Verification items for the finished model (mm, model axes). Round coordinates to 2 decimals unless told otherwise and drop trailing zeros. Write each loop counter-clockwise with the first axis right and the second up, starting at its lowest first coordinate (ties: lowest second). Pieces come first, ordered by that corner, then holes.
from build123d import *

# Parameters (mm, degrees)
SKETCH_W            = 19.36
SKETCH_H            = 103.56
PAD_DEPTH           = 0.8
POCKET_DEPTH        = 5
LINEARPATTERN_COUNT = 6
LINEARPATTERN_PITCH = 16.84


with BuildPart() as part:
    # Sketch → Pad (new body)
    with BuildSketch(Plane.XY):
        with Locations((-9.68, 51.78)):
            Rectangle(SKETCH_W, SKETCH_H)
    extrude(amount=PAD_DEPTH)

    # Sketch001 (on Face6 of Pad) → Pocket (cut)
    with BuildSketch(Plane.XY.offset(0.8)):
        with BuildLine():
            Line((-17.68, 16.68), (-17.68, 2.68))
            ThreePointArc((-17.68, 2.68), (-17.387107, 1.972893), (-16.68, 1.68))
            Line((-16.68, 1.68), (-2.68, 1.68))
            ThreePointArc((-2.68, 1.68), (-1.972893, 1.972893), (-1.68, 2.68))
            Line((-1.68, 2.68), (-1.68, 16.68))
            ThreePointArc((-1.68, 16.68), (-1.972893, 17.387107), (-2.68, 17.68))
            Line((-2.68, 17.68), (-16.68, 17.68))
            ThreePointArc((-16.68, 17.68), (-17.387107, 17.387107), (-17.68, 16.68))
        make_face()
    pocket = extrude(amount=-POCKET_DEPTH, mode=Mode.SUBTRACT)

    # LinearPattern: Pocket ×6
    with Locations(*[(0, i * LINEARPATTERN_PITCH, 0) for i in range(1, LINEARPATTERN_COUNT)]):
        add(pocket, mode=Mode.SUBTRACT)


solid = part.part
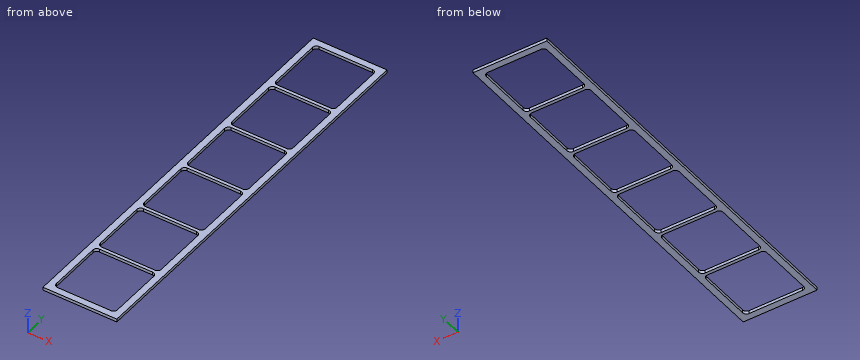
Q1. Sectioned sample at A-A (y = 72). Enter the section's corners in (x, z), plus the area to 3 significant figures.
Recorded:
outline: (-19.36, 0) - (-17.68, 0) - (-17.68, 0.8) - (-19.36, 0.8) - close; (-1.68, 0) - (0, 0) - (0, 0.8) - (-1.68, 0.8) - close
area: 2.69 mm2
Q2. Sectioned sample at C-C (z = 0.3). Give the number of separate pieces and of enclosed holes in the cut face, plus the area to 3 significant figures.
Recorded:
separate pieces: 1
enclosed holes: 6
area: 474 mm2
Q3. Depth check by flat-ended pin: P1, Ø5, axis at x = -4.5, y = 88, coming from the +Z side. Enter the tip coordinate at first touch or a pass-through.
Recorded:
P1: stops at z = 0.8
Q4. Material ranges on line 1 along X through (y, z) = (11.5, 0.6), recorded low to high.
Recorded:
line 1: x = -19.36 to -17.68, -1.68 to 0
Q5. Sectioned sample at B-B (x = -13.25). Enter the section's corners in (y, z), plus the area to 3 significant figures.
Recorded:
outline: (0, 0) - (1.68, 0) - (1.68, 0.8) - (0, 0.8) - close; (17.68, 0) - (18.52, 0) - (18.52, 0.8) - (17.68, 0.8) - close; (34.52, 0) - (35.36, 0) - (35.36, 0.8) - (34.52, 0.8) - close; (51.36, 0) - (52.2, 0) - (52.2, 0.8) - (51.36, 0.8) - close; (68.2, 0) - (69.04, 0) - (69.04, 0.8) - (68.2, 0.8) - close; (85.04, 0) - (85.88, 0) - (85.88, 0.8) - (85.04, 0.8) - close; (101.88, 0) - (103.56, 0) - (103.56, 0.8) - (101.88, 0.8) - close
area: 6.05 mm2
